Model file for the job. Use its own axes, mm. A direction names the side the tool comes from. Give positions to 0.01 mm unless a question says otherwise; leave off trailing zeros. Write each loop counter-clockwise with the first axis right and the second up, starting at its lowest first coordinate (ties: lowest second). Pieces come first, ordered by that corner, then holes.
```python
from build123d import *

# Parameters (mm, degrees)
SKETCH_1_R          = 5
EXTRUDE_1_DEPTH     = 5
SKETCH_3_W          = 5
SKETCH_3_H          = 8
EXTRUDE_2_DEPTH     = 15
SKETCH_2_R          = 2
CUT_EXTRUDE_1_DEPTH = 30
SKETCH_6_W          = 5
SKETCH_6_H          = 8
EXTRUDE_4_DEPTH     = 25
SKETCH_7_W          = 5
SKETCH_7_H          = 8
EXTRUDE_5_DEPTH     = 21
SKETCH_8_W          = 20
SKETCH_8_H          = 20
EXTRUDE_6_DEPTH     = 5
FILLET_2_R          = 2
SKETCH_9_R          = 7.5
CUT_EXTRUDE_3_DEPTH = 5
SKETCH_10_W         = 4
SKETCH_10_H         = 4
EXTRUDE_7_DEPTH     = 5
FILLET_3_R          = 1
FILLET_4_R          = 0.5


with BuildPart() as part:
    # 草图1 → 凸台-拉伸1 (new body)
    with BuildSketch(Plane.XY):
        Circle(SKETCH_1_R)
    extrude(amount=EXTRUDE_1_DEPTH)

    # 草图3 → 凸台-拉伸2 (add)
    with BuildSketch(Plane(origin=(0, 0, 0), x_dir=(0, 0, -1), z_dir=(1, 0, 0))):
        with Locations((-2.5, 0)):
            Rectangle(SKETCH_3_W, SKETCH_3_H)
    extrude(amount=EXTRUDE_2_DEPTH)

    # 草图2 → 切除-拉伸1 (cut)
    with BuildSketch(Plane.XY.offset(5)):
        Circle(SKETCH_2_R)
    extrude(amount=-CUT_EXTRUDE_1_DEPTH, mode=Mode.SUBTRACT)

    # 草图6 → 凸台-拉伸4 (add)
    with BuildSketch(Plane.XY.offset(5)):
        with Locations((12.5, 0)):
            Rectangle(SKETCH_6_W, SKETCH_6_H)
    extrude(amount=EXTRUDE_4_DEPTH)

    # 草图7 → 凸台-拉伸5 (add)
    with BuildSketch(Plane(origin=(15, 0, 0), x_dir=(0, 0, -1), z_dir=(1, 0, 0))):
        with Locations((-27.5, 0)):
            Rectangle(SKETCH_7_W, SKETCH_7_H)
    extrude(amount=EXTRUDE_5_DEPTH)

    # 镜向2: part across plane


with BuildPart() as part_1:
    add(part.part)
    add(part.part.mirror(Plane(origin=(36, 0, 0), x_dir=(0, 0, 1), z_dir=(1, 0, 0))))

    # 草图8 → 凸台-拉伸6 (add)
    with BuildSketch(Plane.XY.offset(30)):
        with Locations((36, 0)):
            Rectangle(SKETCH_8_W, SKETCH_8_H)
    extrude(amount=-EXTRUDE_6_DEPTH)

    # 圆角2
    fillet_2_edges = [part_1.edges().sort_by_distance(p)[0] for p in [
        (26, -10, 27.5),
        (46, 10, 27.5),
        (26, 10, 27.5),
        (46, -10, 27.5),
    ]]
    fillet(fillet_2_edges, radius=FILLET_2_R)

    # 草图9 → 切除-拉伸3 (cut)
    with BuildSketch(Plane.XY.offset(30)):
        with Locations((36, 0)):
            Circle(SKETCH_9_R)
    extrude(amount=-CUT_EXTRUDE_3_DEPTH, mode=Mode.SUBTRACT)

    # 草图10 → 凸台-拉伸7 (add)
    with BuildSketch(Plane.XY.offset(30)):
        with Locations((36, 5.5)):
            Rectangle(SKETCH_10_W, SKETCH_10_H)
        with Locations((41.5, 0)):
            Rectangle(SKETCH_10_W, SKETCH_10_H)
        with Locations((36, -5.5)):
            Rectangle(SKETCH_10_W, SKETCH_10_H)
        with Locations((30.5, 0)):
            Rectangle(SKETCH_10_W, SKETCH_10_H)
    extrude(amount=-EXTRUDE_7_DEPTH)

    # 圆角3
    fillet_3_edges = [part_1.edges().sort_by_distance(p)[0] for p in [
        (34, 3.5, 27.5),
        (38, 3.5, 27.5),
        (39.5, 2, 27.5),
        (39.5, -2, 27.5),
        (38, -3.5, 27.5),
        (34, -3.5, 27.5),
        (32.5, -2, 27.5),
        (32.5, 2, 27.5),
    ]]
    fillet(fillet_3_edges, radius=FILLET_3_R)

    # 圆角4
    fillet_4_edges = [part_1.edges().sort_by_distance(p)[0] for p in [
        (38, 7.228416147, 27.5),
        (34, 7.228416147, 27.5),
        (43.228416147, -2, 27.5),
        (43.228416147, 2, 27.5),
        (34, -7.228416147, 27.5),
        (38, -7.228416147, 27.5),
        (28.771583853, 2, 27.5),
        (28.771583853, -2, 27.5),
    ]]
    fillet(fillet_4_edges, radius=FILLET_4_R)


solid = part_1.part
```
1. Slice it at A-A, the plane y = 0. Write the cut outline in (x, z), and give its area (3 significant figures).
Calculated:
outline: (-5, 0) - (-2, 0) - (-2, 5) - (-5, 5) - close; (2, 0) - (15, 0) - (15, 25) - (32.5, 25) - (32.5, 30) - (10, 30) - (10, 5) - (2, 5) - close; (39.5, 25) - (57, 25) - (57, 0) - (70, 0) - (70, 5) - (62, 5) - (62, 30) - (39.5, 30) - close; (74, 0) - (77, 0) - (77, 5) - (74, 5) - close
area: 585 mm2
2. Pull direction Y, two halves, no side cores. Call faces 6 (the flat face through (34, 6, 28)), 7 (the flat face through (14.6, 4, 16.2)), 8 (the flat face through (62, 0, 17)): +Y half, -Y half, draft (parallel to the pull), parting line (faces both ways), or undercut.
Calculated:
face 6: undercut
face 7: +Y half
face 8: draft
3. Which spindle directions (+Z, -Z, +X, -X, +Y, -Y) get a long thin tool onto all of the face, cutting with end or side? Do faces 1 (the cylindrical face through (26.57, -9.4, 27.46)), 2 (the flat face through (38, -6, 28)), 3 (the flat face through (10, 0, 17)), 4 (the flat face through (59, 4, 16)), 5 (the flat face through (46, -6, 28)). Say none if no direction does.
Calculated:
face 1: +Z, -Z, -X, -Y
face 2: +Z, -Z
face 3: +Z, -X, +Y, -Y
face 4: +Z, -Z, +Y
face 5: +Z, -Z, +X, -Y
4. Pin check, flat tips, straight feed: P1, Ø11, axis at x = 72.5, y = -1, coming from the +Z side; P2, Ø4, axis at y = -6.5, z = 3.5, coming from the +X side; P3, Ø7, axis at x = 14.5, z = 11, coming from the -Y side; P4, Ø2, axis at x = 17, y = 5.5, coming from the -Z side. Stop position of each tip, or through.
Calculated:
P1: stops at z = 5
P2: stops at x = 74.18
P3: stops at y = -4
P4: passes through
5. Slice it at C-C, the plane x = 72. Write the cut outline in (y, z).
Calculated:
outline: (-5, 0) - (-2, 0) - (-2, 5) - (-5, 5) - close; (2, 0) - (5, 0) - (5, 5) - (2, 5) - close
6. Probe probe 1 along Y at (x, z) = (0, 3.9); probe 2 along X at (y, z) = (3.5, 5.5); probe 3 along Z at (x, y) = (43, 8.25). List the from-to ranges inside material, lowest first.
Calculated:
probe 1: y = -5 to -2, 2 to 5
probe 2: x = 10 to 15, 57 to 62
probe 3: z = 25 to 30
7. Slice it at B-B, the plane z = 14.5. Write the cut outline in (x, y), and give its area (3 significant figures).
Calculated:
outline: (10, -4) - (15, -4) - (15, 4) - (10, 4) - close; (57, -4) - (62, -4) - (62, 4) - (57, 4) - close
area: 80.0 mm2
8. Slice it at D-D, the plane x = 58. Write the cut outline in (y, z).
Calculated:
outline: (-4, 0) - (4, 0) - (4, 30) - (-4, 30) - close
